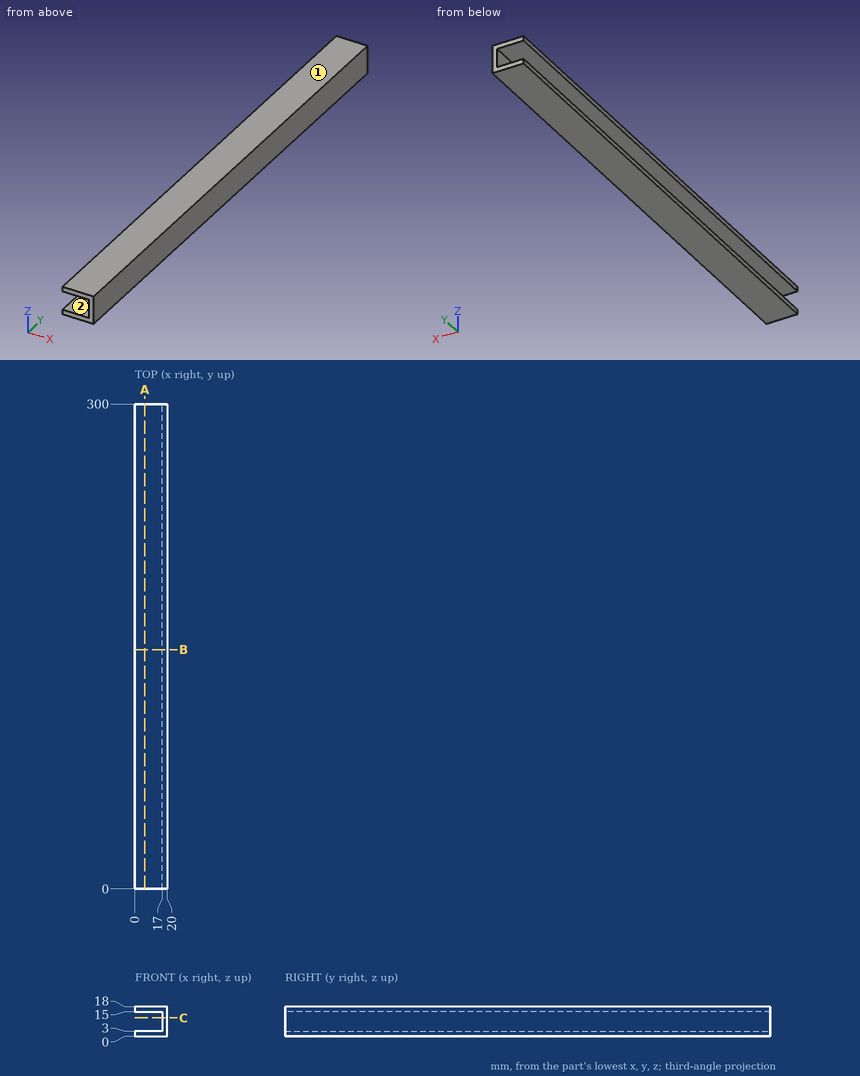
Design review of the part shown in the three views and the two pictorial views. Dimensions are in mm from the part's minimum x, y and z. A direction names the side the tool comes from. Give positions to 0.01 mm unless a question says otherwise; leave off trailing zeros. Loops run counter-clockwise (first coordinate to the right, second up) from the corner with the lowest first, then second, coordinate; pieces in that order, holes last. Notation, with made-up numbers: (57, 61.5) -> (85, 61.5) arc R10 ccw to (85, 79.5) -> close; hole circle Ø6 at (-26, 33). An arc over 180 degrees is marked (long way). Answer as a JSON object with one key per item and string values. Group by question number.
Q1. Tool access review of the marked faces 1 and 2: name each direction out of +Z, -Z, +X, -X, +Y, -Y from which nothing blocks a thin tool from reaching the whole face with its end or side.
Q2. Wall thickness on line 1 along Z through (x, y) = (11.25, 169.5); line 2 along X through (y, z) = (268.5, 3.5): over which ranges is each line inside the solid? List them lowest first.
Q3. Take a section at B-B (y = 148). Write out the cut boundary in (x, z).
Q4. Take a section at A-A (x = 6.25). Write out the cut boundary in (y, z), plus the area to 3 significant figures.
Q5. Take a section at C-C (z = 11.25). Write out the cut boundary in (x, y).
Q6. Insertion check: pin 1 (2 mm diameter, centred on y = 69, z = 3, fed in from -X); pin 2 (9.5 mm diameter, centred on y = 116.5, z = 10, fed in from -X). Each pin has a flat end and moves straight along its axis. Give the tip position at first contact, or say it passes through.
Answer below:
{
 "1": {"face 1": "+Z, +X, -X, +Y, -Y", "face 2": "-X, +Y, -Y"},
 "2": {"line 1": "z = 0 to 3, 15 to 18", "line 2": "x = 17 to 20"},
 "3": {"outline": "(0, 0) -> (20, 0) -> (20, 18) -> (0, 18) -> (0, 15) -> (17, 15) -> (17, 3) -> (0, 3) -> close"},
 "4": {"outline": "(0, 0) -> (300, 0) -> (300, 3) -> (0, 3) -> close; (0, 15) -> (300, 15) -> (300, 18) -> (0, 18) -> close", "area": "1,800 mm2"},
 "5": {"outline": "(17, 0) -> (20, 0) -> (20, 300) -> (17, 300) -> close"},
 "6": {"pin 1": "stops at x = 0", "pin 2": "stops at x = 17"}
}
